Read the model definition and answer for the solid it produces. Units are mm, in the model's axes. Face numbers are marked on the shaded views. A direction names the side the tool comes from. Coordinates: 2 decimals unless noted, no trailing zeros. Write each loop counter-clockwise with the first axis right and the second up, starting at its lowest first coordinate (ties: lowest second). Pieces come first, ordered by that corner, then holes. Notation, with made-up numbers: (-37, 47.5) -> (15, 47.5) arc R20 ccw to (15, 64.5) -> close; hole circle Ø8 at (40.5, -14). An arc over 180 degrees is marked (long way). One line per item, written item: value. Start each with the question number.
1. Find section C-C, the plane y = 66.5. Write down the section's boundary in (x, z), and give its area (3 significant figures).
2. For a pull along Y with two mould halves and no side action, classify the marked faces 5, 6 and 7 as pulls with the +Y half, pulls with the -Y half, needs draft (parallel to the pull), parting line crosses it, or undercut.
3. Find section B-B, the plane x = 70. Write down the section's boundary in (y, z), and give its area (3 significant figures).
4. Consider line 1 along X through (y, z) = (94.5, 12); line 2 along X through (y, z) = (96.5, 3.5); line 3 along Y through (x, z) = (30, 7.75). Determine where each line is inside the solid, lowest interval first.
5. Find section A-A, the plane y = 108.5. Write down the section's boundary in (x, z).
6. Given P1, Ø4, axis at x = 70, z = 10.77, coming from the -Y side; P2, Ø2, axis at x = 16, z = 15, coming from the +Y side; P3, Ø1.5, axis at x = 14.5, z = 11, coming from the +Y side, each flat-ended and moving along its own axis, determine where each tip first touches the part or whether it passes through.
7. For the marked faces 1, 2, 3 and 4, determine the directions among +Z, -Z, +X, -X, +Y, -Y from which every point of the face is accessible in a straight line to the end or side of a thin tool.
8. Find section D-D, the plane y = 81.5. Write down the section's boundary in (x, z).
```python
from build123d import *

# Parameters (mm, degrees)
BOSS_EXTRUDE1_DEPTH = 20
SKETCH2_W           = 20
SKETCH2_H           = 40
CUT_EXTRUDE1_DEPTH  = 142.509716981
SKETCH20_W          = 20
SKETCH20_H          = 20
CUT_EXTRUDE11_DEPTH = 15
SKETCH22_W          = 20
SKETCH22_H          = 20
CUT_EXTRUDE13_DEPTH = 15
SKETCH21_W          = 20
SKETCH21_H          = 20
CUT_EXTRUDE12_DEPTH = 15
SHELL1_START        = 2
SHELL1_DEPTH        = 18
CUT_EXTRUDE10_REACH = 110.167
SKETCH19_R          = 2.5


# Read off the part's stored shape, not the designer's step: Shell1
with BuildPart() as part:
    # Sketch1 → Boss-Extrude1 (new body)
    with BuildSketch(Plane.XY):
        Polygon((58, 114), (58, 115), (80, 115), (80, 20), (60, 0), (0, 0), (-10, 25), (-10, 105), (11, 105), (11, 110), (12, 110), (34, 110), (34, 115), (35, 115), (57, 115), (57, 114), align=None)
    extrude(amount=BOSS_EXTRUDE1_DEPTH)

    # Sketch2 → Cut-Extrude1 (cut, through all)
    with BuildSketch(Plane.XY.offset(20)):
        with Locations((70, 45)):
            Rectangle(SKETCH2_W, SKETCH2_H)
    extrude(amount=-CUT_EXTRUDE1_DEPTH, mode=Mode.SUBTRACT)

    # Sketch20 → Cut-Extrude11 (cut)
    with BuildSketch(Plane(origin=(0, 115, 0), x_dir=(1, 0, 0), z_dir=(0, 1, 0))):
        with Locations((69, -10)):
            Rectangle(SKETCH20_W, SKETCH20_H)
        with Locations((45.5, -10)):
            Rectangle(SKETCH20_W, SKETCH20_H)
    extrude(amount=-CUT_EXTRUDE11_DEPTH, mode=Mode.SUBTRACT)

    # Sketch22 → Cut-Extrude13 (cut)
    with BuildSketch(Plane(origin=(0, 105, 0), x_dir=(1, 0, 0), z_dir=(0, 1, 0))):
        with Locations((1, -10)):
            Rectangle(SKETCH22_W, SKETCH22_H)
    extrude(amount=-CUT_EXTRUDE13_DEPTH, mode=Mode.SUBTRACT)

    # Sketch21 → Cut-Extrude12 (cut)
    with BuildSketch(Plane(origin=(0, 110, 0), x_dir=(1, 0, 0), z_dir=(0, 1, 0))):
        with Locations((24, -10)):
            Rectangle(SKETCH21_W, SKETCH21_H)
    extrude(amount=-CUT_EXTRUDE12_DEPTH, mode=Mode.SUBTRACT)

    # Shell1 outline → Shell1 (cut)
    with BuildSketch(Plane.XY.offset(SHELL1_START)):
        Polygon((58, 20), (58, 70), (78, 70), (78, 98), (36, 98), (36, 93), (13, 93), (13, 88), (-8, 88), (-8, 25.385164807), (1.354065923, 2), (59.171572875, 2), (77.171572875, 20), align=None)
    extrude(amount=SHELL1_DEPTH, mode=Mode.SUBTRACT)

    # Cut-Extrude10: up to this face of the body (flat: up to its plane)
    cut_extrude10_end = Plane(part.part.faces().sort_by_distance((67.585786438, 20, 11))[0])
    # Sketch19 → Cut-Extrude10 (cut, up to the picked face)
    with BuildSketch(Plane(origin=(0, 70, 0), x_dir=(1, 0, 0), z_dir=(0, 1, 0)), mode=Mode.PRIVATE) as cut_extrude10_sk1:
        with Locations(Location((70, -10.774964387, 0), (0, 0, 270))):
            Circle(SKETCH19_R)
    cut_extrude10_tool1 = split(extrude(cut_extrude10_sk1.sketch, amount=-CUT_EXTRUDE10_REACH, mode=Mode.PRIVATE), bisect_by=cut_extrude10_end, keep=Keep.BOTH, mode=Mode.PRIVATE)
    add(cut_extrude10_tool1.solids().sort_by(Axis((70, 70, 10.774964), (0, -1, 0)))[0], mode=Mode.SUBTRACT)


solid = part.part
```
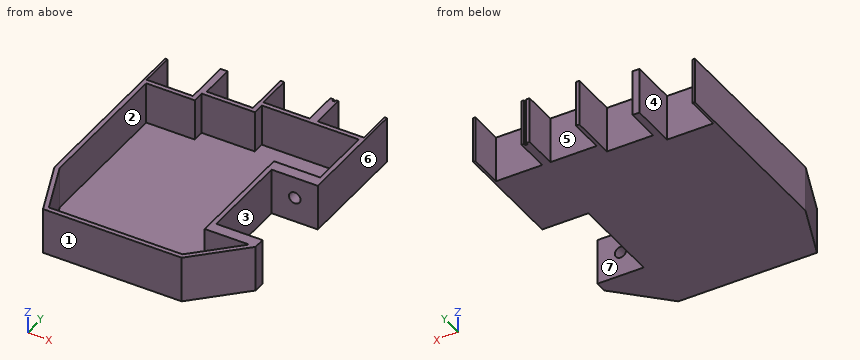
Answer block:
1. outline: (-10, 0) -> (80, 0) -> (80, 20) -> (58, 20) -> (58, 2) -> (-8, 2) -> (-8, 20) -> (-10, 20) -> close; hole circle Ø5 at (70, 10.77)
1. area: 592 mm2
2. face 5: pulls with the +Y half
2. face 6: needs draft
2. face 7: undercut
3. outline: (10, 0) -> (25, 0) -> (25, 8.27) -> (20, 8.27) -> (20, 2) -> (12.83, 2) -> (12.83, 20) -> (10, 20) -> close; (20, 13.27) -> (25, 13.27) -> (25, 20) -> (20, 20) -> close; (65, 0) -> (100, 0) -> (100, 20) -> (98, 20) -> (98, 2) -> (70, 2) -> (70, 8.27) -> (65, 8.27) -> close; (65, 13.27) -> (70, 13.27) -> (70, 20) -> (65, 20) -> close
3. area: 317 mm2
4. line 1: x = -10 to -9, 11 to 36, 78 to 80
4. line 2: x = -10 to -9, 11 to 14, 34 to 36, 78 to 80
4. line 3: y = 0 to 2, 93 to 95
5. outline: (11, 0) -> (14, 0) -> (14, 20) -> (11, 20) -> close; (34, 0) -> (35.5, 0) -> (35.5, 20) -> (34, 20) -> close; (55.5, 0) -> (59, 0) -> (59, 20) -> (55.5, 20) -> close; (79, 0) -> (80, 0) -> (80, 20) -> (79, 20) -> close
6. P1: stops at y = 8
6. P2: stops at y = 95
6. P3: stops at y = 110
7. face 1: +Z, -Z, +X, -X, -Y
7. face 2: +Z
7. face 3: +Z, -Z, +X
7. face 4: +Z, -Z, +Y
8. outline: (-10, 0) -> (80, 0) -> (80, 20) -> (78, 20) -> (78, 2) -> (-8, 2) -> (-8, 20) -> (-10, 20) -> close
